Here's the drawing with two shaded views (mm, measured from the low corner). I have some questions. Coordinates: 2 decimals unless noted, no trailing zeros. Loops run counter-clockwise (first coordinate to the right, second up) from the corner with the lowest first, then second, coordinate; pieces in that order, holes last. Notation, with made-up numbers: (-22.75, 25) - (1.25, 25) arc R24 ccw to (1.25, 39) - close; hole circle Ø8 at (27.25, 2). An arc over 180 degrees is marked (long way). Use a Markdown table: item, result.
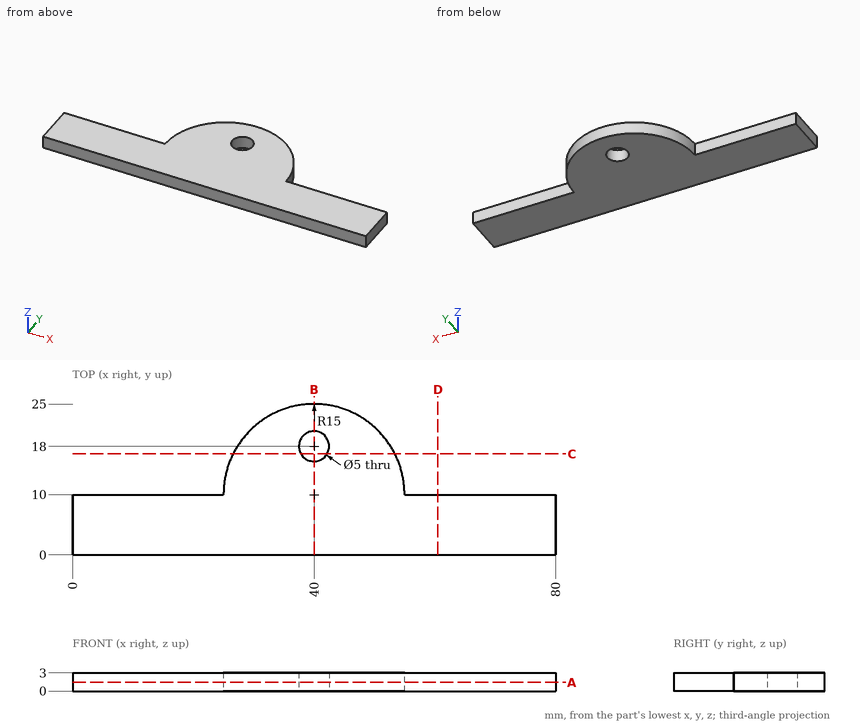
Q1. I want a section at B-B, the plane x = 40. Write out the boundary of the cut face in (y, z).
Check values:
| item | result |
|---|---|
| outline | (0, 0) - (15.5, 0) - (15.5, 3) - (0, 3) - close; (20.5, 0) - (25, 0) - (25, 3) - (20.5, 3) - close |
Q2. I want a section at C-C, the plane y = 16.75. Write out the boundary of the cut face in (x, z).
Check values:
| item | result |
|---|---|
| outline | (26.6, 0) - (37.83, 0) - (37.83, 3) - (26.6, 3) - close; (42.17, 0) - (53.4, 0) - (53.4, 3) - (42.17, 3) - close |
Q3. I want a section at A-A, the plane z = 1.45. Write out the boundary of the cut face in (x, y), then the cut area to 3 significant figures.
Check values:
| item | result |
|---|---|
| outline | (0, 0) - (80, 0) - (80, 10) - (55, 10) arc R15 ccw to (25, 10) - (0, 10) - close; hole circle Ø5 at (40, 18) |
| area | 1,130 mm^2 |
Q4. Please list where these lines run through material, in increasing order: L1, parallel to Y at x = 40, z = 1.2; L2, parallel to Y at x = 12.5, z = 2.3; L3, parallel to Y at x = 41, z = 0.35. Write a range as from..to.
Check values:
| item | result |
|---|---|
| L1 | 0..15.5, 20.5..25 |
| L2 | 0..10 |
| L3 | 0..15.71, 20.29..24.97 |
Q5. Will these pins go through, and if not, where does the flat tip stop? P1, Ø4.5, axis at x = 40, y = 18, coming from the -Z side; P2, Ø0.9, axis at x = 14, z = 1, coming from the +Y side; P3, Ø1.5, axis at y = 15, z = 1.5, coming from the -X side.
Check values:
| item | result |
|---|---|
| P1 | through |
| P2 | y = 10 |
| P3 | x = 25.61 |
Q6. I want a section at D-D, the plane x = 60.5. Write out the boundary of the cut face in (y, z).
Check values:
| item | result |
|---|---|
| outline | (0, 0) - (10, 0) - (10, 3) - (0, 3) - close |
